The drawing under review shows one solid part. Ordinate dimensions are in mm from its lowest x, y, z. Coordinates: 2 decimals unless noted, no trailing zeros. Order: outer loops, then holes, each group sorted by start corner. A loop starts at its lowest first (then second) coordinate and runs counter-clockwise, first axis right, second up. Notation, with made-up numbers: (23.5, 50.25) - (81.5, 50.25) arc R33 cw to (81.5, 89.25) - close; hole circle Ø10 at (26, 13.25). An arc over 180 degrees is marked (long way). Answer in a Markdown table with one row per item.
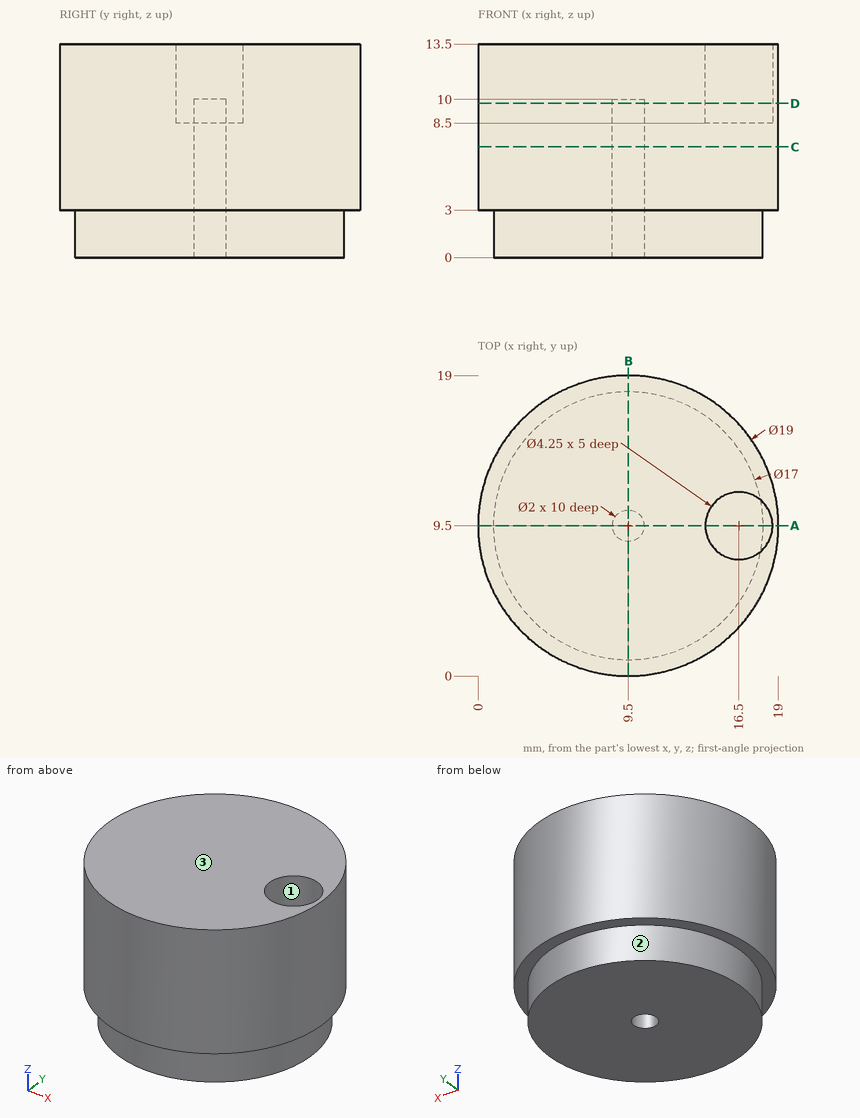
Item 1: Clearance check with flat-ended pins moving along their axes: pin 1 Ø0.6 at (x, y) = (9.5, 9) entering from -Z; pin 2 Ø4 at (x, y) = (16.5, 9.5) entering from +Z; pin 3 Ø1 at (y, z) = (12, 8) entering from +X; pin 4 Ø6 at (y, z) = (8.5, 5.5) entering from -X. State where each tip first meets the part, or that it passes through.
Check values:
| item | result |
|---|---|
| pin 1 | z = 10 |
| pin 2 | z = 8.5 |
| pin 3 | x = 18.79 |
| pin 4 | x = 0 |
Item 2: We need section B-B, the plane x = 9.5. Write out the cut boundary in (y, z), then the cut area to 4 significant figures.
Check values:
| item | result |
|---|---|
| outline | (0, 3) - (1, 3) - (1, 0) - (8.5, 0) - (8.5, 10) - (10.5, 10) - (10.5, 0) - (18, 0) - (18, 3) - (19, 3) - (19, 13.5) - (0, 13.5) - close |
| area | 230.5 mm^2 |
Item 3: To check wall thickness, follow line 1 (Y direction, x = 9.5, z = 3.75); line 2 (Z direction, x = 18, y = 12.25); line 3 (Y direction, x = 16.5, z = 10.5) (3 decimals). State the ranges of each line that lie inside material, in increasing order. Write a range as from..to.
Check values:
| item | result |
|---|---|
| line 1 | 0..8.5, 10.5..19 |
| line 2 | 3..13.5 |
| line 3 | 3.077..7.375, 11.625..15.923 |
Item 4: We need section A-A, the plane y = 9.5. Write out the cut boundary in (x, z) (3 decimals).
Check values:
| item | result |
|---|---|
| outline | (0, 3) - (1, 3) - (1, 0) - (8.5, 0) - (8.5, 10) - (10.5, 10) - (10.5, 0) - (18, 0) - (18, 3) - (19, 3) - (19, 13.5) - (18.625, 13.5) - (18.625, 8.5) - (14.375, 8.5) - (14.375, 13.5) - (0, 13.5) - close |
Item 5: We need section D-D, the plane z = 9.75. Write out the cut boundary in (x, y) (3 decimals).
Check values:
| item | result |
|---|---|
| outline | circle Ø19 at (9.5, 9.5); hole circle Ø2 at (9.5, 9.5); hole circle Ø4.25 at (16.5, 9.5) |
Item 6: We need section C-C, the plane z = 7. Write out the cut boundary in (x, y), then the cut area to 3 significant figures.
Check values:
| item | result |
|---|---|
| outline | circle Ø19 at (9.5, 9.5); hole circle Ø2 at (9.5, 9.5) |
| area | 280 mm^2 |
Item 7: Mouldability with a two-part tool opening along X and no side actions: class the marked faces 1, 2 and 3 as +X half, -X half, draft (parallel to the pull), parting line (faces both ways), or undercut.
Check values:
| item | result |
|---|---|
| face 1 | undercut |
| face 2 | parting line |
| face 3 | draft |
